Autodesk Inventor part; units mm, degrees
ref_plane "YZ Plane" through (0, 0, 0) normal (1, 0, 0) x (0, 1, 0)
ref_plane "XZ Plane" through (0, 0, 0) normal (0, 1, 0) x (-1, 0, 0)
ref_plane "XY Plane" through (0, 0, 0) normal (0, 0, 1) x (1, 0, 0)
sketch "Sketch1" plane through (0, 0, 0) normal (0, 1, 0) x (-1, 0, 0)
  circle A0 centre (0, 0) radius 19.75
  circle A1 centre (0, 0) radius 5
  circle A2 centre (0, 16.6) radius 1.1
  circle A3 centre (16.6, 0) radius 1.1
  circle A4 centre (0, -16.6) radius 1.1
  circle A5 centre (-16.6, 0) radius 1.1
  circle A6 centre (-7.6, 0) radius 1.1
  circle A7 centre (0, 7.6) radius 1.1
  circle A8 centre (7.6, 0) radius 1.1
  circle A9 centre (0, -7.6) radius 1.1
  point P0 (0, 19.75)
  point P1 (19.75, 0)
  point P2 (0, -19.75)
  point P3 (-19.75, 0)
  point P4 (0, -5)
  point P5 (-5, 0)
  point P6 (0, 5)
  point P7 (5, 0)
  dimension "d0" = 39.5
  dimension "d1" = 10
  dimension "d2" = 2.2
  dimension "d3" = 3.15
  dimension "d4" = 2.2
  dimension "d5" = 3.15
  dimension "d6" = 2.2
  dimension "d7" = 3.15
  dimension "d8" = 2.2
  dimension "d9" = 3.15
  dimension "d10" = 2.2
  dimension "d11" = 2.2
  dimension "d12" = 2.2
  dimension "d13" = 2.2
  dimension "d14" = 2.6
  dimension "d15" = 2.6
  dimension "d16" = 2.6
  dimension "d17" = 2.6
extrude "Extrusion1" add sketch "Sketch1" along normal blind 5
sketch "Sketch2" plane through (0, 5, 0) normal (0, 1, 0) x (1, 0, 0)
  line L0 (17.6777, 17.6777) -> (67.6777, 17.6777) construction
  line L1 (0, 0) -> (-35.3553, -35.3553)
  line L2 (0, 0) -> (50, 0) construction
  circle A0 centre (-35.3553, -35.3553) radius 2.75
  circle A1 centre (0, 0) radius 19.75
  line L3 (13.9654, -13.9654) -> (-13.9654, 13.9654)
  line L4 (-13.9654, 13.9654) -> (-56.3918, -28.461)
  line L5 (13.9654, -13.9654) -> (-28.461, -56.3918)
  line L6 (-28.461, -56.3918) -> (-56.3918, -28.461)
  circle A2 centre (0, -16.6) radius 1.1
  circle A3 centre (0, -16.6) radius 1.1
  circle A4 centre (0, -7.6) radius 1.1
  circle A5 centre (0, -7.6) radius 1.1
  circle A6 centre (-7.6, 0) radius 1.1
  circle A7 centre (-7.6, 0) radius 1.1
  circle A8 centre (-16.6, 0) radius 1.1
  circle A9 centre (-16.6, 0) radius 1.1
  circle A10 centre (0, 0) radius 5
  dimension "d22" = 50
  dimension "d23" = 135
  dimension "d24" = 5.5
  dimension "d25" = 60
  dimension "d26" = 60
extrude "Extrusion2" add sketch "Sketch2" against normal blind 5 contours A1 L5 L6 L4
sketch "Sketch3" plane through (0, 5, 0) normal (0, 1, 0) x (1, 0, 0)
  line L0 (-28.461, -56.3918) -> (-56.3918, -28.461)
  arc A0 (13.9654, -13.9654) -> (-13.9654, 13.9654) centre (0, 0) ccw
  line L1 (-28.461, -56.3918) -> (13.9654, -13.9654)
  spline S0 degree 2 poles (-13.9654, 13.9654) (-84.8528, -84.8528) (13.9654, -13.9654) knots 0 0 0 1 1 1
  line L2 (13.9654, -13.9654) -> (-28.461, -56.3918)
  line L3 (-56.3918, -28.461) -> (-13.9654, 13.9654)
  point P0 (-42.4264, -42.4264)
extrude "Extrusion3" cut sketch "Sketch3" against normal blind 5 contours L0 S0 L1 | L0 L3 S0
properties part number "Servo-head.finalV1"
Input: part model. Units: mm. Frame: model coordinates. Coordinates: 2 decimals unless noted, no trailing zeros. Use a Markdown table: item, result.
1) Pull-direction query (X, two-part tool) for faces 1 (the flat face through (-14, 5, 15)), 2 (the cylindrical face through (0.14, 2.46, -17.69)), 3 (the cylindrical face through (13.655, 2.465, -14.269)); classes: released by +X, released by -X, zero draft, split by the parting line, or undercut.
Results found:
| item | result |
|---|---|
| face 1 | zero draft |
| face 2 | undercut |
| face 3 | split by the parting line |
2) Contact query for flat-ended pins moving along their axis: pin 1 (1 mm diameter, centred on y = 2, z = -12.5, fed in from -X); pin 2 (2 mm diameter, centred on y = 3.5, z = 22, fed in from +X); pin 3 (3 mm diameter, centred on y = 1, z = 20.5, fed in from -X). Output: stop coordinate, or through.
Results found:
| item | result |
|---|---|
| pin 1 | stops at x = -15.37 |
| pin 2 | stops at x = 3.97 |
| pin 3 | stops at x = -37.32 |
3) Material intervals for line 1 along Z through (x, y) = (0, 2.3); line 2 along X through (y, z) = (0.75, 37); line 3 along X through (y, z) = (2.35, -3.5), sorted ascending. Write a range as from..to.
Results found:
| item | result |
|---|---|
| line 1 | z = -19.75..-17.7, -15.5..-8.7, -6.5..-5, 5..6.5, 8.7..15.5, 17.7..23.71 |
| line 2 | x = -43.4..-37.56, -33.15..-21.41 |
| line 3 | x = -21.32..-3.57, 3.57..19.44 |
4) Cut plane A-A (z = 0). Give the number of separate pieces and of enclosed holes in the cut face, then the cut area to 3 significant figures.
Results found:
| item | result |
|---|---|
| separate pieces | 6 |
| enclosed holes | 0 |
| area | 123 mm2 |
